from build123d import *

# Parameters (mm, degrees)
F0_R     = 5.7
F0_R_2   = 11.2
F1_DEPTH = 7
F2_R     = 5


with BuildPart() as f1:
    # F0 (on Top) → F1 (new body)
    with BuildSketch(Plane.XY):
        Polygon((14.950241, -10.861986), (61.069731, 0), (14.950241, 10.861986), (18.871585, 58.080765), (-5.710484, 17.575063), (-49.40645, 35.895887), (-18.479514, 0), (-49.40645, -35.895887), (-5.710484, -17.575063), (18.871585, -58.080765), align=None)
        with Locations((-24.27051, -17.633558)):
            Circle(F0_R, mode=Mode.SUBTRACT)
        with BuildLine():
            Line((9.27051, -10.490836), (9.27051, -20.77537))
            ThreePointArc((9.27051, -20.77537), (6.873673, -21.154992), (4.711456, -22.256696))
            Line((4.711456, -22.256696), (-1.333641, -13.936334))
            ThreePointArc((-1.333641, -13.936334), (4.326238, -13.314791), (9.27051, -10.490836))
        make_face(mode=Mode.SUBTRACT)
        with BuildLine():
            Line((-7.112633, -12.058626), (-16.893806, -15.236721))
            ThreePointArc((-16.893806, -15.236721), (-17.995511, -13.074504), (-19.711456, -11.358558))
            Line((-19.711456, -11.358558), (-13.666359, -3.038196))
            ThreePointArc((-13.666359, -3.038196), (-11.326238, -8.228994), (-7.112633, -12.058626))
        make_face(mode=Mode.SUBTRACT)
        Circle(F0_R_2, mode=Mode.SUBTRACT)
        with Locations((9.27051, -28.531695)):
            Circle(F0_R, mode=Mode.SUBTRACT)
        with BuildLine():
            ThreePointArc((22.623296, 2.396836), (22.243675, 0), (22.623296, -2.396836))
            Line((22.623296, -2.396836), (12.842123, -5.574932))
            ThreePointArc((12.842123, -5.574932), (14, 0), (12.842123, 5.574932))
            Line((12.842123, 5.574932), (22.623296, 2.396836))
        make_face(mode=Mode.SUBTRACT)
        with Locations((30, 0)):
            Circle(F0_R, mode=Mode.SUBTRACT)
        with Locations((-24.27051, 17.633558)):
            Circle(F0_R, mode=Mode.SUBTRACT)
        with BuildLine():
            Line((-13.666359, 3.038196), (-19.711456, 11.358558))
            ThreePointArc((-19.711456, 11.358558), (-17.995511, 13.074504), (-16.893806, 15.236721))
            Line((-16.893806, 15.236721), (-7.112633, 12.058626))
            ThreePointArc((-7.112633, 12.058626), (-11.326238, 8.228994), (-13.666359, 3.038196))
        make_face(mode=Mode.SUBTRACT)
        with BuildLine():
            Line((9.27051, 20.77537), (9.27051, 10.490836))
            ThreePointArc((9.27051, 10.490836), (4.326238, 13.314791), (-1.333641, 13.936334))
            Line((-1.333641, 13.936334), (4.711456, 22.256696))
            ThreePointArc((4.711456, 22.256696), (6.873673, 21.154992), (9.27051, 20.77537))
        make_face(mode=Mode.SUBTRACT)
        with Locations((9.27051, 28.531695)):
            Circle(F0_R, mode=Mode.SUBTRACT)
    extrude(amount=F1_DEPTH)

    # F2
    f2_edges = [f1.edges().sort_by_distance(p)[0] for p in [
        (18.871585, -58.080765, 3.5),
        (61.069731, 0, 3.5),
        (18.871585, 58.080765, 3.5),
        (-49.40645, 35.895887, 3.5),
        (-49.40645, -35.895887, 3.5),
    ]]
    fillet(f2_edges, radius=F2_R)


solid = f1.part
For this review, take the finished solid that the model builds, in its own axes (mm). A direction names the side the tool comes from. Round coordinates to 2 decimals unless told otherwise and drop trailing zeros. Loops run counter-clockwise (first coordinate to the right, second up) from the corner with the lowest first, then second, coordinate; pieces in that order, holes last. Notation, with made-up numbers: (-29.75, -12.5) - (21.25, -12.5) arc R20 cw to (21.25, 17.5) - close; hole circle Ø2 at (30.25, 33.25). An arc over 180 degrees is marked (long way). One line per question, with ' | ' between items.
Q1. Take a section at B-B (y = -32). Give the boundary of the cut face in (x, z).
Taken from the geometry:
outline: (3.04, 0) - (4.75, 0) - (4.75, 7) - (3.04, 7) - close; (13.79, 0) - (16.71, 0) - (16.71, 7) - (13.79, 7) - close
Q2. For pin 1 (10.5 mm diameter, centred on x = -24.27, y = 17.63, fed in from +Z); pin 2 (1 mm diameter, centred on x = 33.5, z = 1, fed in from +Y); pin 3 (2 mm diameter, centred on y = -14, z = 2.5, fed in from -X); pin 4 (2 mm diameter, centred on y = 11, z = 2, fed in from -X), all flat-tipped, find the tip position at first contact; note any pin that passes through.
Taken from the geometry:
pin 1: passes through | pin 2: stops at y = 6.61 | pin 3: stops at x = -31.4 | pin 4: stops at x = -28.82
Q3. Tool access review of faces 4 (the flat face through (16.048, -24.075, 3.451)), 5 (the cylindrical face through (6.906, -21.145, 3.451)), 6 (the flat face through (-27.13, 10.04, 3.45)): name each direction out of +Z, -Z, +X, -X, +Y, -Y from which nothing blocks a thin tool from reaching the whole face with its end or side.
Taken from the geometry:
face 4: +Z, -Z, +X | face 5: +Z, -Z | face 6: +Z, -Z, -X
Q4. Take a section at C-C (z = 5.5). State how many separate pieces and enclosed holes the cut face has, and give its area (3 significant figures).
Taken from the geometry:
separate pieces: 1 | enclosed holes: 11 | area: 1,710 mm²
Q5. For line 1 along X through (y, z) = (1, 1.25); line 2 along X through (y, z) = (-27.5, 3); line 3 along Y through (x, z) = (-1, 2.75), list the stretches that pass through material, from the lowest coordinate up. Write a range as [from, to].
Taken from the geometry:
line 1: x = [-19.34, -11.16], [11.16, 13.96], [22.31, 24.39], [35.61, 44.16] | line 2: x = [-34.09, -29.38], [0.31, 3.66], [14.88, 16.33] | line 3: y = [-25.34, -14.4], [-13.96, -11.16], [11.16, 13.96], [14.4, 25.34]
Q6. Take a section at A-A (x = 0). Give the boundary of the cut face in (y, z).
Taken from the geometry:
outline: (-26.98, 0) - (-15.77, 0) - (-15.77, 7) - (-26.98, 7) - close; (-14, 0) - (-11.2, 0) - (-11.2, 7) - (-14, 7) - close; (11.2, 0) - (14, 0) - (14, 7) - (11.2, 7) - close; (15.77, 0) - (26.98, 0) - (26.98, 7) - (15.77, 7) - close
Q7. The part is to be moulded in two halves that separate along Y. For faces 1 (the cylindrical face through (44.26, -0.09, 3.55)), 2 (the flat face through (-17.6, 22.56, 3.45)), 3 (the cylindrical face through (-11.19, 0.49, 3.45)), say which applies: released by +Y, released by -Y, zero draft, split by the parting line, or undercut.
Taken from the geometry:
face 1: split by the parting line | face 2: released by +Y | face 3: undercut
